Autodesk Fusion 360 part; units mm, degrees
sketch "Sketch1" plane through (0, 0, 0) normal (0, 0, 1) x (1, 0, 0)
  circle A0 centre (0, 0) radius 29.75
  circle A1 centre (0, 0) radius 18.925
  line L0 (0, 0) -> (0, 29.75) construction
  circle A2 centre (-7.5, 22) radius 2
  circle A3 centre (7.5, 22) radius 2
  line L1 (0, -18.419) -> (2, -18.419)
  line L2 (2, -18.419) -> (2, -18.819)
  line L3 (0, -18.925) -> (0, -18.419) construction
  line L4 (-2, -18.419) -> (-2, -18.819)
  line L5 (0, -18.419) -> (-2, -18.419)
  line L6 (16.9513, 7.4775) -> (17.2978, 7.6775)
  line L7 (15.9513, 9.2095) -> (16.9513, 7.4775)
  line L8 (15.9513, 9.2095) -> (14.9513, 10.9416)
  line L9 (14.9513, 10.9416) -> (15.2978, 11.1416)
  line L10 (-14.9513, 10.9416) -> (-15.2978, 11.1416)
  line L11 (-15.9513, 9.2095) -> (-14.9513, 10.9416)
  line L12 (-15.9513, 9.2095) -> (-16.9513, 7.4775)
  line L13 (-16.9513, 7.4775) -> (-17.2978, 7.6775)
  dimension "d1" = 59.5
  dimension "d78" = 37.85
  dimension "d131" = 4
  dimension "d132" = 7.5
  dimension "d135" = 2
  dimension "d136" = 0.4
  dimension "d138" = 360
extrude "Extrude16" add sketch "Sketch1" along normal blind 4 contours A0 | A1 L6 L7 L8 L9 | A1 L1 L2 L4 L5 | A1 L10 L11 L12 L13 | A2 | A3
extrude "Extrude17" cut sketch "Sketch1" along normal blind 4 contours A2 | A3
Design review of the part built by this model. Coordinates are the model's own, in mm. A direction names the side the tool comes from. Round coordinates to 2 decimals unless told otherwise and drop trailing zeros. Write each loop counter-clockwise with the first axis right and the second up, starting at its lowest first coordinate (ties: lowest second). Pieces come first, ordered by that corner, then holes. Notation, with made-up numbers: (83.25, -8.5) - (126.25, -8.5) arc R28 ccw to (126.25, 19.5) - close; hole circle Ø6 at (79.5, -33). An arc over 180 degrees is marked (long way). Return JSON: item names as keys, results as strings. Group by question number.
Item 1: We need section D-D on z = 1.6. Give the number of separate pieces and of enclosed holes in the cut face, and give its area (3 significant figures).
Item 2: For probe 1 along Y at (x, z) = (-7.5, 2.45); probe 2 along Y at (x, z) = (12, 3.45); probe 3 along Y at (x, z) = (4.5, 1.1), list the stretches that pass through material, from the lowest coordinate up. Write a range as [from, to].
Item 3: The part is to be moulded in two halves that separate along X. For faces 1 (the face through (16.51, -9.25, 1.97)), 2 (the face through (15.993, -25.085, 1.972)), 3 (the face through (0, -19, 4)), say which applies: pulls with the +X half, pulls with the -X half, needs draft (parallel to the pull), parting line crosses it, or undercut.
Item 4: Insertion check: P1, Ø1.5, axis at y = 18, z = 3, coming from the +X side; P2, Ø1, axis at x = 13, z = 2, coming from the +Y side; P3, Ø1, axis at x = -23.5, z = 0.5, coming from the -Y side. Each pin has a flat end and moves straight along its axis. Give the tip position at first contact, or say it passes through.
Item 5: We need section B-B on x = 0. Write out the cut boundary in (y, z) (3 decimals), and give its area (3 significant figures).
Item 6: We need section C-C on y = 22. Write out the cut boundary in (x, z).
Item 7: We need section A-A on y = 0. Write out the cut boundary in (x, z) (3 decimals), and give its area (3 significant figures).
Item 8: Machinability: for faces 4 (the face through (0, -18.419, 2)), 5 (the face through (0, -19, 0)), which of the approach directions +Z, -Z, +X, -X, +Y, -Y give a long, thin tool a straight path to every point of the face, cutting with its end or side? Answer none if there is none.
Model answer:
{
 "1": {"separate pieces": "1", "enclosed holes": "3", "area": "1,640 mm²"},
 "2": {"probe 1": "y = [-28.79, -17.38], [17.38, 20], [24, 28.79]", "probe 2": "y = [-27.22, -14.63], [14.63, 27.22]", "probe 3": "y = [-29.41, -18.38], [18.38, 29.41]"},
 "3": {"face 1": "undercut", "face 2": "parting line crosses it", "face 3": "needs draft"},
 "4": {"P1": "stops at x = 24.24", "P2": "stops at y = 27", "P3": "stops at y = -18.87"},
 "5": {"outline": "(-29.75, 0) - (-18.419, 0) - (-18.419, 4) - (-29.75, 4) - close; (18.925, 0) - (29.75, 0) - (29.75, 4) - (18.925, 4) - close", "area": "88.6 mm²"},
 "6": {"outline": "(-20.03, 0) - (-9.5, 0) - (-9.5, 4) - (-20.03, 4) - close; (-5.5, 0) - (5.5, 0) - (5.5, 4) - (-5.5, 4) - close; (9.5, 0) - (20.03, 0) - (20.03, 4) - (9.5, 4) - close"},
 "7": {"outline": "(-29.75, 0) - (-18.925, 0) - (-18.925, 4) - (-29.75, 4) - close; (18.925, 0) - (29.75, 0) - (29.75, 4) - (18.925, 4) - close", "area": "86.6 mm²"},
 "8": {"face 4": "+Z, -Z", "face 5": "-Z, +X, -X, +Y, -Y"}
}
